Work out the finished part from the listing and answer in its coordinate system (mm). A direction names the side the tool comes from. Give positions to 0.01 mm unless a question says otherwise; leave off trailing zeros. Order: outer loops, then holes, each group sorted by start corner. A loop starts at its lowest first (then second) coordinate and runs counter-clockwise, first axis right, second up.
```python
from build123d import *

# Parameters (mm, degrees)
SKETCH_1_W          = 30
SKETCH_1_H          = 30
EXTRUDE_1_DEPTH     = 3
SKETCH_2_W          = 30
SKETCH_2_H          = 3
EXTRUDE_2_DEPTH     = 8
EXTRUDE_3_DEPTH     = 2
SKETCH_4_R          = 1.5
CUT_EXTRUDE_1_DEPTH = 32.906112399


with BuildPart() as part:
    # 草图1 → 凸台-拉伸1 (new body)
    with BuildSketch(Plane.XY):
        Rectangle(SKETCH_1_W, SKETCH_1_H)
    extrude(amount=EXTRUDE_1_DEPTH)

    # 草图2 → 凸台-拉伸2 (add)
    with BuildSketch(Plane(origin=(0, 0, 0), x_dir=(-1, 0, 0), z_dir=(0, 0, -1))):
        with Locations((0, -13.5)):
            Rectangle(SKETCH_2_W, SKETCH_2_H)
    extrude(amount=EXTRUDE_2_DEPTH)

    # 草图3 → 凸台-拉伸3 (add)
    with BuildSketch(Plane(origin=(0, 0, 0), x_dir=(-1, 0, 0), z_dir=(0, 0, -1))):
        with BuildLine():
            Line((-2.305106483, 11.311404977), (-2.027743838, 11.566704685))
            add(Edge.make_bspline(
                [(-2.027743838, 11.566704685), (-1.794878972, 11.457790237), (-1.355574197, 11.252320696), (-0.747856089, 10.942285903), (-0.229982958, 10.649795688), (0.194428064, 10.374755127), (0.533566886, 10.121882158), (0.77438392, 9.881751463), (0.944974603, 9.664968691), (1.015639241, 9.391415806), (0.9966854, 9.097589735), (0.941039457, 8.786331398), (0.817795551, 8.5236158), (0.633519261, 8.332982487), (0.449181288, 8.195889891), (0.302760924, 8.088135642), (0.197092176, 8.017364927), (0.134764911, 7.999081008), (0.112361118, 7.992508778)],
                knots=[0, 0, 0, 0, 2.197927662, 4.146439677, 5.832238005, 7.279845715, 8.471106398, 9.436605479, 10.191661816, 10.788881907, 11.804124267, 12.685011878, 13.484502328, 14.241053406, 14.92571184, 15.446805523, 15.80115196, 16, 16, 16, 16], degree=3))
            add(Edge.make_bspline(
                [(0.112361118, 7.992508778), (0.050011554, 8.002947143), (-0.08737732, 8.02594835), (-0.259956516, 8.196857468), (-0.416014276, 8.442101169), (-0.49556336, 8.644926258), (-0.540071468, 8.758407901)],
                knots=[0, 0, 0, 0, 0.700838763, 1.544316304, 2.626032788, 4, 4, 4, 4], degree=3))
            add(Edge.make_bspline(
                [(-0.540071468, 8.758407901), (-0.5821962, 8.852359749), (-0.669510424, 9.047098852), (-0.824057914, 9.340433436), (-1.009761281, 9.641406724), (-1.212425661, 9.95948938), (-1.451127048, 10.280678596), (-1.709872913, 10.617383427), (-1.996269827, 10.962872749), (-2.200425668, 11.193269267), (-2.305106483, 11.311404977)],
                knots=[0, 0, 0, 0, 0.792668784, 1.643007677, 2.550308334, 3.515107773, 4.545787362, 5.629874198, 6.784719067, 8, 8, 8, 8], degree=3))
        make_face()
        with BuildLine():
            Line((-10.673263566, 7.822308973), (6.806886784, 7.822308973))
            Line((6.806886784, 7.822308973), (8.294559155, 9.183907414))
            Line((8.294559155, 9.183907414), (10.340108664, 7.311709558))
            Line((10.340108664, 7.311709558), (-7.697918825, 7.311709558))
            add(Edge.make_bspline(
                [(-7.697918825, 7.311709558), (-7.881871988, 7.308656331), (-8.247237029, 7.302592056), (-8.789546429, 7.25479995), (-9.319932334, 7.173180033), (-9.666114906, 7.095155579), (-9.838023782, 7.056409851)],
                knots=[0, 0, 0, 0, 1.02169224, 2.029269967, 3.021366146, 4, 4, 4, 4], degree=3))
            Line((-9.838023782, 7.056409851), (-10.673263566, 7.822308973))
        make_face()
        with BuildLine():
            Line((-4.073293347, 6.801110143), (-2.399661931, 5.439511702))
            Line((-2.399661931, 5.439511702), (-3.329457162, 5.184211995))
            add(Edge.make_bspline(
                [(-3.329457162, 5.184211995), (-3.661918376, 4.911100535), (-4.308266223, 4.38013633), (-5.275377087, 3.641671086), (-6.20188694, 2.972304041), (-7.094304982, 2.384361746), (-7.944987667, 1.862571734), (-8.76101121, 1.42223379), (-9.537567982, 1.049381648), (-10.053055168, 0.85340936), (-10.301345473, 0.759017063)],
                knots=[0, 0, 0, 0, 1.244563663, 2.419593658, 3.519436122, 4.550355101, 5.510468856, 6.405273195, 7.231881577, 8, 8, 8, 8], degree=3))
            Line((-10.301345473, 0.759017063), (-10.39590092, 1.014316771))
            add(Edge.make_bspline(
                [(-10.39590092, 1.014316771), (-10.017360387, 1.257610495), (-9.271761863, 1.736817941), (-8.210938681, 2.507364265), (-7.222105067, 3.311601244), (-6.458376899, 4.010201777), (-5.891338542, 4.563771343), (-5.510356994, 4.954154228), (-5.169522327, 5.319561824), (-4.868268622, 5.659752471), (-4.609963017, 5.977639283), (-4.390692723, 6.270958293), (-4.211876273, 6.540564482), (-4.117256895, 6.718455576), (-4.073293347, 6.801110143)],
                knots=[0, 0, 0, 0, 1.874567547, 3.692272479, 5.459531722, 7.182386108, 8.002686949, 8.761086549, 9.454870534, 10.08449878, 10.653979193, 11.160886839, 11.610118005, 12, 12, 12, 12], degree=3))
        make_face()
        with BuildLine():
            Line((2.157910627, 6.205410825), (2.343869674, 6.545810435))
            add(Edge.make_bspline(
                [(2.343869674, 6.545810435), (2.605834901, 6.436341272), (3.112201517, 6.224742464), (3.838791155, 5.904957081), (4.5109758, 5.606334574), (5.126868337, 5.32410298), (5.683835605, 5.050933425), (6.18816715, 4.801822938), (6.633579267, 4.564873458), (7.024336582, 4.343514345), (7.367605722, 4.13296053), (7.659729552, 3.917895038), (7.913118437, 3.70773837), (8.117652642, 3.493912706), (8.281765506, 3.281612264), (8.390719488, 3.064564894), (8.468546645, 2.849731388), (8.476569277, 2.703294503), (8.480518201, 2.631214919)],
                knots=[0, 0, 0, 0, 1.812650006, 3.50376826, 5.068178675, 6.508778607, 7.828769435, 9.028683626, 10.099947299, 11.049250256, 11.896072215, 12.668859108, 13.363683509, 13.994673249, 14.555440601, 15.068439001, 15.541464367, 16, 16, 16, 16], degree=3))
            add(Edge.make_bspline(
                [(8.480518201, 2.631214919), (8.476404976, 2.582724581), (8.467267846, 2.475007981), (8.423484243, 2.297731425), (8.344229944, 2.09247344), (8.25102173, 1.867292552), (8.147973226, 1.655779591), (8.0404517, 1.495783125), (7.940944184, 1.382250748), (7.860971901, 1.362739725), (7.828085615, 1.354716381)],
                knots=[0, 0, 0, 0, 0.783511922, 1.740496043, 2.929679364, 4.326021141, 5.673987734, 6.697847245, 7.464527372, 8, 8, 8, 8], degree=3))
            add(Edge.make_bspline(
                [(7.828085615, 1.354716381), (7.778254634, 1.363823494), (7.665304798, 1.384466213), (7.508869781, 1.514426132), (7.33907668, 1.700823102), (7.236160537, 1.861095257), (7.178804877, 1.950415698)],
                knots=[0, 0, 0, 0, 0.659298193, 1.494404119, 2.603619392, 4, 4, 4, 4], degree=3))
            add(Edge.make_bspline(
                [(7.178804877, 1.950415698), (7.05077175, 2.120334623), (6.790528866, 2.465715476), (6.351980668, 2.957201814), (5.879949473, 3.445544273), (5.448204004, 3.838103862), (5.071308787, 4.156382587), (4.753669197, 4.410381652), (4.40326017, 4.679131769), (4.018624623, 4.958216125), (3.602200666, 5.252417066), (3.150171333, 5.557368175), (2.666341418, 5.878628105), (2.330498068, 6.094484039), (2.157910627, 6.205410825)],
                knots=[0, 0, 0, 0, 1.156150992, 2.350017333, 3.577869138, 4.847260874, 5.520054583, 6.25951119, 7.058018181, 7.920529522, 8.842772332, 9.829688202, 10.884692641, 12, 12, 12, 12], degree=3))
        make_face()
        with BuildLine():
            Line((4.852740874, 2.546115016), (3.922945643, 2.120615504))
            add(Edge.make_bspline(
                [(3.922945643, 2.120615504), (3.778143809, 1.82421938), (3.495891085, 1.246473844), (3.04537482, 0.421735242), (2.600207435, -0.348814984), (2.14910532, -1.060375348), (1.693094833, -1.712036898), (1.235082828, -2.306624664), (0.778013133, -2.84595086), (0.454910586, -3.169143954), (0.298320165, -3.325778259)],
                knots=[0, 0, 0, 0, 1.204096835, 2.347067039, 3.429841553, 4.452343735, 5.421672099, 6.332275, 7.191743416, 8, 8, 8, 8], degree=3))
            add(Edge.make_bspline(
                [(0.298320165, -3.325778259), (0.467371652, -3.460680933), (0.804829073, -3.729971132), (1.331492998, -4.10738687), (1.88197699, -4.447975474), (2.445743055, -4.770543562), (3.033662777, -5.053897321), (3.636746234, -5.318574444), (4.26028991, -5.550228819), (4.903129981, -5.75541281), (5.562944375, -5.935964084), (6.244219172, -6.082699716), (6.942165498, -6.206022022), (7.660409719, -6.300592633), (8.396506838, -6.36624034), (9.152451449, -6.40361966), (9.926304872, -6.414121821), (10.448350425, -6.397679491), (10.712026756, -6.38937475)],
                knots=[0, 0, 0, 0, 0.934343793, 1.865119626, 2.797078927, 3.729977298, 4.669861379, 5.615133413, 6.574575313, 7.542078903, 8.529761733, 9.528696818, 10.55179032, 11.591106972, 12.657506233, 13.743698561, 14.860380514, 16, 16, 16, 16], degree=3))
            Line((10.712026756, -6.38937475), (10.712026756, -6.644674457))
            add(Edge.make_bspline(
                [(10.712026756, -6.644674457), (10.593551143, -6.694413754), (10.368009945, -6.789102106), (10.057143895, -6.952034998), (9.783930664, -7.117072932), (9.551528569, -7.293653878), (9.360617359, -7.47996839), (9.209175094, -7.673945806), (9.097776051, -7.877179087), (9.057887744, -8.021061239), (9.03839534, -8.091372801)],
                knots=[0, 0, 0, 0, 1.342228497, 2.555191034, 3.66432754, 4.674491749, 5.598393505, 6.443878379, 7.239562799, 8, 8, 8, 8], degree=3))
            add(Edge.make_bspline(
                [(9.03839534, -8.091372801), (8.782895007, -8.053774011), (8.278227338, -7.979508381), (7.534842543, -7.847534784), (6.814769096, -7.696310098), (6.119241864, -7.525795044), (5.446927157, -7.340877009), (4.800151359, -7.136303868), (4.178578687, -6.9112148), (3.578469668, -6.672573488), (3.001920816, -6.414512859), (2.449407864, -6.137513581), (1.922822868, -5.839647417), (1.417450221, -5.528897707), (0.937404482, -5.197825017), (0.484023103, -4.846060424), (0.04937862, -4.482669543), (-0.220108602, -4.221530185), (-0.354112421, -4.091677381)],
                knots=[0, 0, 0, 0, 1.193225404, 2.35687475, 3.487949324, 4.592342887, 5.665273416, 6.709260648, 7.725799817, 8.71919469, 9.692664653, 10.643553074, 11.573847077, 12.487217793, 13.384029152, 14.266643611, 15.138080182, 16, 16, 16, 16], degree=3))
            add(Edge.make_bspline(
                [(-0.354112421, -4.091677381), (-0.687954777, -4.336238901), (-1.36469164, -4.831993238), (-2.457220721, -5.491503236), (-3.616311833, -6.105133202), (-4.849137014, -6.663426184), (-6.155501273, -7.164833907), (-7.532331542, -7.620724798), (-8.982918656, -8.017005113), (-9.979873138, -8.235475251), (-10.487304519, -8.346672508)],
                knots=[0, 0, 0, 0, 0.895891654, 1.816075456, 2.760633746, 3.735148952, 4.745060468, 5.78983574, 6.875067292, 8, 8, 8, 8], degree=3))
            Line((-10.487304519, -8.346672508), (-10.581859967, -8.006272898))
            add(Edge.make_bspline(
                [(-10.581859967, -8.006272898), (-10.110834321, -7.868872221), (-9.183269378, -7.598296613), (-7.83804971, -7.122751604), (-6.554032396, -6.606440296), (-5.334681224, -6.042862661), (-4.178464198, -5.435332451), (-3.08902742, -4.779483566), (-2.056181335, -4.088247104), (-1.415110101, -3.578144674), (-1.097948607, -3.325778259)],
                knots=[0, 0, 0, 0, 1.105387851, 2.176779602, 3.213352566, 4.222748287, 5.202262626, 6.154710299, 7.087067382, 8, 8, 8, 8], degree=3))
            add(Edge.make_bspline(
                [(-1.097948607, -3.325778259), (-1.260055043, -3.106837933), (-1.589883827, -2.661372453), (-2.048484783, -1.948011623), (-2.492442326, -1.18834854), (-2.920242442, -0.381785035), (-3.331401412, 0.471478138), (-3.720806012, 1.374691494), (-4.095894147, 2.32503193), (-4.327447855, 2.979277785), (-4.44521144, 3.312014139)],
                knots=[0, 0, 0, 0, 0.875624334, 1.781583235, 2.724691925, 3.703827006, 4.716008585, 5.76891757, 6.865316105, 8, 8, 8, 8], degree=3))
            Line((-4.44521144, 3.312014139), (-4.073293347, 3.397114042))
            add(Edge.make_bspline(
                [(-4.073293347, 3.397114042), (-3.933134319, 3.09897675), (-3.657432916, 2.512522417), (-3.221796476, 1.660810191), (-2.775613682, 0.850452935), (-2.31503743, 0.084755389), (-1.845304898, -0.639422738), (-1.362545341, -1.320629255), (-0.870186722, -1.961636505), (-0.524078683, -2.362851182), (-0.354112421, -2.559879136)],
                knots=[0, 0, 0, 0, 1.121804492, 2.206658228, 3.257157778, 4.27140299, 5.248867787, 6.195889759, 7.114040017, 8, 8, 8, 8], degree=3))
            add(Edge.make_bspline(
                [(-0.354112421, -2.559879136), (-0.192509947, -2.36144819), (0.135702757, -1.958437299), (0.582016589, -1.299215138), (1.007149635, -0.591689341), (1.404711522, 0.170425626), (1.772606892, 0.985808869), (2.115397305, 1.853872388), (2.43500954, 2.774833691), (2.620849746, 3.412007893), (2.715787766, 3.737513652)],
                knots=[0, 0, 0, 0, 0.869716896, 1.76638467, 2.70366274, 3.675080695, 4.68700289, 5.743663211, 6.847331519, 8, 8, 8, 8], degree=3))
            Line((2.715787766, 3.737513652), (4.852740874, 2.546115016))
        make_face()
    extrude(amount=EXTRUDE_3_DEPTH)

    # 草图4 → 切除-拉伸1 (cut, through all)
    with BuildSketch(Plane(origin=(0, -12, 0), x_dir=(1, 0, 0), z_dir=(0, 1, 0))):
        with Locations(Location((-10, 3.999978925, 0), (0, 0, 180))):
            Circle(SKETCH_4_R)
        with Locations((10, 3.999978925)):
            Circle(SKETCH_4_R)
    extrude(amount=-CUT_EXTRUDE_1_DEPTH, mode=Mode.SUBTRACT)


solid = part.part
```
1. The mould has two halves that part along X. Classify faces 5 (the face through (0, -15, -2)), 6 (the face through (15, -4, 1)), 7 (the face through (2.858, 5.314, -0.986)), 8 (the face through (-8.89, -13.48, -2.99)): pulls with the +X half, pulls with the -X half, needs draft (parallel to the pull), parting line crosses it, or undercut.
Findings below:
face 5: needs draft
face 6: pulls with the +X half
face 7: undercut
face 8: undercut
2. The part is cut by section A-A (z = -3). Write down the section's boundary in (x, y), then the cut area to 3 significant figures.
Findings below:
outline: (-15, -15) - (-11.12, -15) - (-11.12, -12) - (-15, -12) - close; (-8.88, -15) - (8.88, -15) - (8.88, -12) - (-8.88, -12) - close; (11.12, -15) - (15, -15) - (15, -12) - (11.12, -12) - close
area: 76.6 mm2
3. Which of the six approach directions +Z, -Z, +X, -X, +Y, -Y give full straight-line access (tool end or side, diameter ignored) to faces 1 (the face through (-1, 7.312, -1)), 2 (the face through (-9.303, 8.261, -0.986)), 3 (the face through (-0.66, 7.65, -2)), 4 (the face through (0, -12, -4))?
Findings below:
face 1: -Z, -X
face 2: -Z, -X, +Y
face 3: -Z, +X, -X, +Y
face 4: -Z, +X, -X
4. Given P1, Ø1.1, axis at x = -3, y = 8, coming from the -Z side; P2, Ø1, axis at x = -8, z = -3, coming from the +Y side; P3, Ø3.5, axis at x = -5, y = -3, coming from the -Z side; P4, Ø2.5, axis at x = -10, z = -4, coming from the -Y side, each flat-ended and moving along its own axis, determine where each tip first touches the part or whether it passes through.
Findings below:
P1: stops at z = -2
P2: stops at y = -12
P3: stops at z = 0
P4: passes through
5. The part is cut by section C-C (z = -6.75). Write down the section's boundary in (x, y), then the cut area to 3 significant figures.
Findings below:
outline: (-15, -15) - (15, -15) - (15, -12) - (-15, -12) - close
area: 90.0 mm2
6. The part is cut by section D-D (y = -13). Write down the section's boundary in (x, z), then the cut area to 3 significant figures.
Findings below:
outline: (-15, -8) - (15, -8) - (15, 3) - (-15, 3) - close; hole circle Ø3 at (-10, -4); hole circle Ø3 at (10, -4)
area: 316 mm2
7. The part is cut by section B-B (x = -12.5). Write down the section's boundary in (y, z).
Findings below:
outline: (-15, -8) - (-12, -8) - (-12, 0) - (15, 0) - (15, 3) - (-15, 3) - close
8. Straight lines are drawn through the part: probe 1 along Y at (x, z) = (-10, -0.5); probe 2 along Y at (x, z) = (9, -0.75); probe 3 along Z at (x, y) = (-10, -13). For each, find the intervals that lie inside material, in ascending order.
Findings below:
probe 1: y = -15 to -12, -6.99 to -6.41, 7.31 to 7.62
probe 2: y = -15 to -12, -8.01 to -7.52, 1.31 to 1.94, 7.22 to 7.82
probe 3: z = -8 to -5.5, -2.5 to 3
